For this review, take the finished solid that the model builds, in its own axes (mm). A direction names the side the tool comes from. Give positions to 0.01 mm unless a question says otherwise; leave off trailing zeros. Order: outer loops, then holes, each group sorted by start corner. A loop starts at its lowest first (then second) coordinate and runs counter-clockwise, first axis right, second up.
Item 1: The part is to be moulded in two halves that separate along Z. For faces 1 (the flat face through (5, -7, 5.7)), 2 (the cylindrical face through (-1.73, 7.81, 8.88)), 3 (the cylindrical face through (-1.73, 7.81, 2.81)), say which applies: released by +Z, released by -Z, zero draft, split by the parting line, or undercut.
Item 2: Machinability: for faces 4 (the cylindrical face through (7.715, -4.919, 6.562)), 5 (the flat face through (2, -8, 11.9)), 6 (the flat face through (2, -8, 10.4)), which of the approach directions +Z, -Z, +X, -X, +Y, -Y give a long, thin tool a straight path to every point of the face, cutting with its end or side? Answer none if there is none.
Item 3: Consider section B-B (z = 6.5). Give the boundary of the cut face in (x, y).
Item 4: Consider section A-A (x = 0). Give the boundary of the cut face in (y, z).
Item 5: For P1, Ø8, axis at x = 6.5, y = 5.5, coming from the +Z side; P2, Ø5, axis at y = 6, z = 5.5, coming from the -X side; P3, Ø3, axis at y = 2, z = 3.5, coming from the +X side; P4, Ø4, axis at y = -2, z = 6, coming from the -X side, all flat-tipped, find the tip position at first contact; note any pin that passes through.
Item 6: For probe 1 along Z at (x, y) = (-2, -8.5); probe 2 along Z at (x, y) = (-9.5, 1.75); probe 3 along X at (y, z) = (5, 11.5), list the stretches that pass through material, from the lowest coordinate up.
Item 7: Consider section C-C (y = 5). Give the boundary of the cut face in (x, z) (3 decimals).
Item 8: Consider section D-D (z = 1.75). Give the boundary of the cut face in (x, y).
Solid Edge part; units mm, degrees
sketch "Sketch1" plane through (0, 0, 0) normal (0, 0, 1) x (1, 0, 0)
  circle A0 centre (0, 0) radius 8
extrude "Protrusion1" add sketch "Sketch1" along normal blind 16.2
sketch "Sketch2" plane through (0, 0, 7.4) normal (0, 0, 1) x (0, -1, 0)
  circle A0 centre (0, 0) radius 9.15
extrude "ExtrudedProtrusion_2" add sketch "Sketch2" against normal blind 1.7
sketch "Sketch3" plane through (0, 0, 10.4) normal (0, 0, 1) x (0, -1, 0)
  line L0 (0, 10.9697) -> (-9.5, 5.4848)
  line L1 (-9.5, 5.4848) -> (-9.5, -5.4848)
  line L2 (-9.5, -5.4848) -> (0, -10.9697)
  line L3 (0, -10.9697) -> (9.5, -5.4848)
  line L4 (9.5, -5.4848) -> (9.5, 5.4848)
  line L5 (9.5, 5.4848) -> (0, 10.9697)
extrude "ExtrudedProtrusion_3" add sketch "Sketch3" along normal blind 1.5
Resolved:
1. face 1: released by -Z
1. face 2: undercut
1. face 3: zero draft
2. face 4: -Z
2. face 5: +Z
2. face 6: none
3. outline: circle Ø18.3 at (0, 0)
4. outline: (-9.5, 10.4) - (-8, 10.4) - (-8, 7.4) - (-9.15, 7.4) - (-9.15, 5.7) - (-8, 5.7) - (-8, 0) - (8, 0) - (8, 5.7) - (9.15, 5.7) - (9.15, 7.4) - (8, 7.4) - (8, 10.4) - (9.5, 10.4) - (9.5, 11.9) - (8, 11.9) - (8, 16.2) - (-8, 16.2) - (-8, 11.9) - (-9.5, 11.9) - close
5. P1: stops at z = 16.2
5. P2: stops at x = -8.45
5. P3: stops at x = 7.98
5. P4: stops at x = -9.15
6. probe 1: z = 5.7 to 7.4, 10.4 to 11.9
6. probe 2: z = 10.4 to 11.9
6. probe 3: x = -8.08 to 8.08
7. outline: (-8.083, 10.4) - (-6.245, 10.4) - (-6.245, 7.4) - (-7.663, 7.4) - (-7.663, 5.7) - (-6.245, 5.7) - (-6.245, 0) - (6.245, 0) - (6.245, 5.7) - (7.663, 5.7) - (7.663, 7.4) - (6.245, 7.4) - (6.245, 10.4) - (8.083, 10.4) - (8.083, 11.9) - (6.245, 11.9) - (6.245, 16.2) - (-6.245, 16.2) - (-6.245, 11.9) - (-8.083, 11.9) - close
8. outline: circle Ø16 at (0, 0)
